```python
from build123d import *

# Parameters (mm, degrees)
SKETCH4_R          = 5.8
SKETCH4_R_2        = 5.4825
CUT_EXTRUDE2_DEPTH = 8
CUT_EXTRUDE1_DEPTH = 8
CIRPATTERN1_COUNT  = 18


with BuildPart() as part:
    # Sketch1 → Revolve1 (revolve)
    with BuildSketch(Plane.XY, mode=Mode.PRIVATE) as revolve1_sk:
        with BuildLine():
            Line((-1.6, 4), (9.6, 4))
            Line((9.6, 4), (9.6, 7.2))
            ThreePointArc((9.6, 7.2), (8.8, 8), (8, 7.2))
            Line((8, 7.2), (8, 5.55))
            Line((8, 5.55), (0, 5.55))
            Line((0, 5.55), (0, 7.2))
            ThreePointArc((0, 7.2), (-0.8, 8), (-1.6, 7.2))
            Line((-1.6, 7.2), (-1.6, 4))
        make_face()
    revolve(revolve1_sk.sketch.rotate(Axis((-1.6, 0, 0), (1, 0, 0)), 90), axis=Axis((-1.6, 0, 0), (1, 0, 0)))

    # Sketch4 → Cut-Extrude2 (cut)
    with BuildSketch(Plane(origin=(0, 0, 0), x_dir=(0, 0, -1), z_dir=(1, 0, 0))):
        Circle(SKETCH4_R)
        Circle(SKETCH4_R_2, mode=Mode.SUBTRACT)
    extrude(amount=CUT_EXTRUDE2_DEPTH, mode=Mode.SUBTRACT)

    # Sketch3 → Cut-Extrude1 (cut)
    with BuildSketch(Plane(origin=(0, 0, 0), x_dir=(0, 0, -1), z_dir=(1, 0, 0))):
        with BuildLine():
            Line((-0.642345316, 5.604560113), (-0.343021997, 4.962659182))
            Line((-0.343021997, 4.962659182), (0.343021997, 4.962659182))
            Line((0.343021997, 4.962659182), (0.642345316, 5.604560113))
            ThreePointArc((0.642345316, 5.604560113), (0, 5.64125), (-0.642345316, 5.604560113))
        make_face()
    cut_extrude1 = extrude(amount=CUT_EXTRUDE1_DEPTH, mode=Mode.SUBTRACT)

    # CirPattern1: Cut-Extrude1 ×18 about axis
    cirpattern1_axis = Axis((0, 0, 0), (1, 0, 0))
    for i in range(1, CIRPATTERN1_COUNT):
        add(cut_extrude1.rotate(cirpattern1_axis, i * 360 / CIRPATTERN1_COUNT), mode=Mode.SUBTRACT)


solid = part.part
```
Could you check a few things on this model? Use its own coordinates, in mm. A direction names the side the tool comes from. Round coordinates to 2 decimals unless told otherwise and drop trailing zeros. Loops run counter-clockwise (first coordinate to the right, second up) from the corner with the lowest first, then second, coordinate; pieces in that order, holes last. Notation, with made-up numbers: (8, -33.75) - (28, -33.75) arc R15 cw to (28, -9.75) - close; hole circle Ø4 at (-3.5, 14). An arc over 180 degrees is marked (long way). Use CSV: the item, a comma, the result in double quotes.
Item 1: If we section it at C-C on x = -0.5: List the corners of the cut face in (y, z) for me, then the cut area to 3 significant figures.
Here are the results:
outline,"circle Ø15.88 at (0, 0); hole circle Ø8 at (0, 0)"
area,"148 mm²"
Item 2: If we section it at B-B on y = 0: List the corners of the cut face in (x, z) for me, then the cut area to 3 significant figures.
Here are the results:
outline,"(-1.6, -7.2) arc R0.8 ccw to (0, -7.2) - (0, -5.48) - (8, -5.48) - (8, -7.2) arc R0.8 ccw to (9.6, -7.2) - (9.6, -4) - (-1.6, -4) - close; (-1.6, 4) - (9.6, 4) - (9.6, 7.2) arc R0.8 ccw to (8, 7.2) - (8, 5.48) - (0, 5.48) - (0, 7.2) arc R0.8 ccw to (-1.6, 7.2) - close"
area,"48.2 mm²"
Item 3: If we mould it in two halves opening along X, with no side actions, what happens to faces 1 (the flat face through (0, 5, 2)), 2 (the cylindrical face through (4.078, 3.905, -0.867)), 3 (the flat face through (9.6, 3, -3))? For each: pulls with the +X half, pulls with the -X half, needs draft (parallel to the pull), parting line crosses it, or undercut.
Here are the results:
face 1,"undercut"
face 2,"needs draft"
face 3,"pulls with the +X half"
Item 4: If we section it at A-A on z = 0: List the corners of the cut face in (x, y) for me.
Here are the results:
outline,"(-1.6, -7.2) arc R0.8 ccw to (0, -7.2) - (0, -4.96) - (8, -4.96) - (8, -7.2) arc R0.8 ccw to (9.6, -7.2) - (9.6, -4) - (-1.6, -4) - close; (-1.6, 4) - (9.6, 4) - (9.6, 7.2) arc R0.8 ccw to (8, 7.2) - (8, 4.96) - (0, 4.96) - (0, 7.2) arc R0.8 ccw to (-1.6, 7.2) - close"
Item 5: I need wall thicknesses on L1, parallel to Y at x = 2.25, z = 0; L2, parallel to X at y = 6, z = -1; L3, parallel to Y at x = 1.5, z = 3.5. Which ranges of each line are inside material? Lowest first, please. Write a range as [from, to].
Here are the results:
L1,"y = [-4.96, -4], [4, 4.96]"
L2,"x = [-1.6, 0], [8, 9.6]"
L3,"y = [-3.6, -1.94], [1.94, 3.6]"
Item 6: Will these pins go through, and if not, where does the flat tip stop? pin 1 (6.5 mm diameter, centred on y = 0, z = 0, fed in from -X); pin 2 (5 mm diameter, centred on x = 1.5, y = -3.5, fed in from +Z); pin 3 (0.5 mm diameter, centred on x = 2.5, z = 0, fed in from -Y); pin 4 (6 mm diameter, centred on y = 4.5, z = 6.5, fed in from +X).
Here are the results:
pin 1,"passes through"
pin 2,"stops at z = 7.69"
pin 3,"stops at y = -4.96"
pin 4,"stops at x = 9.6"
Item 7: For faces 4 (the flat face through (-1.6, 3, 3)), 5 (the flat face through (8, 5, -2)), which set-ups out of +Z, -Z, +X, -X, +Y, -Y let a thin tool reach every point of the face, with its end or its side?
Here are the results:
face 4,"+Z, -Z, -X, +Y, -Y"
face 5,"none"
